```python
from build123d import *

# Parameters (mm, degrees)
SKETCH014_W   = 84.5
SKETCH014_H   = 109
SKETCH014_W_2 = 78.5
SKETCH014_H_2 = 103
PAD006_DEPTH  = 17
FILLET002_R   = 3
FILLET004_R   = 2.5


with BuildPart() as part:
    # Sketch014 → Pad006 (new body)
    with BuildSketch(Plane.XY):
        with Locations((4.75, 6.5)):
            Rectangle(SKETCH014_W, SKETCH014_H)
        with Locations((4.75, 6.5)):
            Rectangle(SKETCH014_W_2, SKETCH014_H_2, mode=Mode.SUBTRACT)
    extrude(amount=-PAD006_DEPTH)

    # Fillet002
    fillet002_edges = [part.edges().sort_by_distance(p)[0] for p in [
        (-34.5, 58, -8.5),
        (-34.5, -45, -8.5),
        (44, 58, -8.5),
        (44, -45, -8.5),
    ]]
    fillet(fillet002_edges, radius=FILLET002_R)

    # Fillet004
    fillet004_edges = [part.edges().sort_by_distance(p)[0] for p in [
        (47, 61, -8.5),
        (-37.5, 61, -8.5),
        (47, -48, -8.5),
        (-37.5, -48, -8.5),
        (-37.5, 6.5, 0),
        (4.75, -48, 0),
        (47, 6.5, 0),
        (4.75, 61, 0),
    ]]
    fillet(fillet004_edges, radius=FILLET004_R)


with BuildPart() as part_1:
    # Body005 placement: moved
    add(part.part.moved(Location((0, 0, 4.5))))


solid = part_1.part
```
Input: part model. Units: mm. Frame: model coordinates. A direction names the side the tool comes from. Give positions to 0.01 mm unless a question says otherwise; leave off trailing zeros. Order: outer loops, then holes, each group sorted by start corner. A loop starts at its lowest first (then second) coordinate and runs counter-clockwise, first axis right, second up.
1. Reachability of faces 1 (the cylindrical face through (5, -47, 4)), 2 (the flat face through (4, -45, -4)) from +Z, -Z, +X, -X, +Y, -Y: full face, straight path, thin tool, end or side. Return the list, or none.
Derived:
face 1: +Z, +X, -X, -Y
face 2: +Z, -Z
2. Mould query, pull axis Y, two halves, no side actions, for faces 3 (the flat face through (-36, 7, -12.5)), 4 (the flat face through (4, 58, -4)), 5 (the flat face through (4, 61, -5)). Classes: released by +Y, released by -Y, zero draft, split by the parting line, or undercut.
Derived:
face 3: zero draft
face 4: undercut
face 5: released by +Y
3. Section A-A on y = -39.5. Return the cut outline in (x, z).
Derived:
outline: (-37.5, -12.5) - (-34.5, -12.5) - (-34.5, 4.5) - (-35, 4.5) arc R2.5 ccw to (-37.5, 2) - close; (44, -12.5) - (47, -12.5) - (47, 2) arc R2.5 ccw to (44.5, 4.5) - (44, 4.5) - close
4. Section C-C on z = -2.25. Return the cut outline in (x, y).
Derived:
outline: (-37.5, -45.5) arc R2.5 ccw to (-35, -48) - (44.5, -48) arc R2.5 ccw to (47, -45.5) - (47, 58.5) arc R2.5 ccw to (44.5, 61) - (-35, 61) arc R2.5 ccw to (-37.5, 58.5) - close; hole (-34.5, -42) arc R3 ccw to (-31.5, -45) - (41, -45) arc R3 ccw to (44, -42) - (44, 55) arc R3 ccw to (41, 58) - (-31.5, 58) arc R3 ccw to (-34.5, 55) - close
5. Section B-B on x = 20. Return the cut outline in (y, z), and give its area (3 significant figures).
Derived:
outline: (-48, -12.5) - (-45, -12.5) - (-45, 4.5) - (-45.5, 4.5) arc R2.5 ccw to (-48, 2) - close; (58, -12.5) - (61, -12.5) - (61, 2) arc R2.5 ccw to (58.5, 4.5) - (58, 4.5) - close
area: 99.3 mm2
6. Material intervals for L1, parallel to Y at x = 15.5, z = -1.75; L2, parallel to X at y = 22, z = 1.5; L3, parallel to X at y = -9, z = 3.75, sorted ascending.
Derived:
L1: y = -48 to -45, 58 to 61
L2: x = -37.5 to -34.5, 44 to 47
L3: x = -36.79 to -34.5, 44 to 46.29
